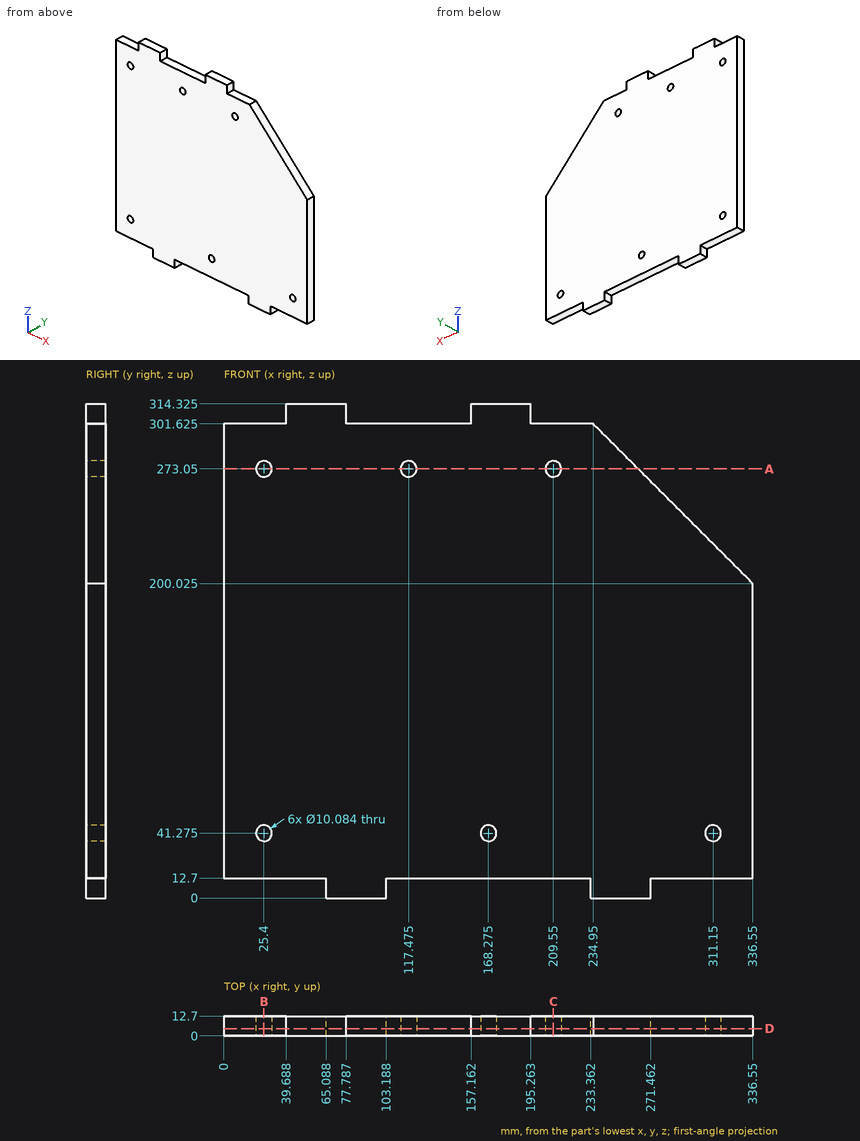
Here's the drawing with two shaded views (mm, measured from the low corner). I have some questions. Round coordinates to 2 decimals unless told otherwise and drop trailing zeros. Write each loop counter-clockwise with the first axis right and the second up, starting at its lowest first coordinate (ties: lowest second). Pieces come first, ordered by that corner, then holes. Notation, with made-up numbers: M -0.75,26 L 32.25,26 A14 cw 32.25,41 Z; hole C 80,17.5 d11. An arc over 180 degrees is marked long. Answer in a Markdown table with one row per item. Add a question column.
Q1. Imagine slicing it at D-D (y = 4.75). Give the number of separate pieces and of enclosed holes in the cut face, then the cut area to 3 significant figures.
Q2. Imagine slicing it at C-C (x = 209.55). Please give me the cut outline in (y, z) (1 decimal).
Q3. Will these pins go through, and if not, where does the flat tip stop? pin 1 Ø4 at (y, z) = (8.5, 3.5) entering from -X; pin 2 Ø4 at (y, z) = (9.5, 9) entering from +X; pin 3 Ø6 at (x, z) = (209.55, 273.05) entering from +Y; pin 4 Ø1.5 at (x, y) = (79, 10.5) entering from +Z (1 decimal).
Q4. Imagine slicing it at B-B (x = 25.4). Please give me the cut outline in (y, z) (1 decimal).
Q5. If I drill on line 1 (Z direction, x = 133.5, y = 9.25) (1 decimal); line 2 (X direction, y = 8.25, z = 273.05) (1 decimal); line 3 (Z direction, x = 311.15, y = 4.25) (1 decimal), over which ranges is the centre line in solid material (lowest first)? Write a range as from..to.
Q6. Imagine slicing it at A-A (z = 273.05). Please give me the cut outline in (x, y) (1 decimal).
Values:
| question | item | result |
|---|---|---|
| 1 | separate pieces | 1 |
| 1 | enclosed holes | 6 |
| 1 | area | 93,500 mm^2 |
| 2 | outline | M 0,12.7 L 12.7,12.7 L 12.7,268 L 0,268 Z; M 0,278.1 L 12.7,278.1 L 12.7,301.6 L 0,301.6 Z |
| 3 | pin 1 | x = 65.09 |
| 3 | pin 2 | x = 271.46 |
| 3 | pin 3 | through |
| 3 | pin 4 | z = 301.6 |
| 4 | outline | M 0,12.7 L 12.7,12.7 L 12.7,36.2 L 0,36.2 Z; M 0,46.3 L 12.7,46.3 L 12.7,268 L 0,268 Z; M 0,278.1 L 12.7,278.1 L 12.7,301.6 L 0,301.6 Z |
| 5 | line 1 | 12.7..301.6 |
| 5 | line 2 | 0..20.4, 30.4..112.4, 122.5..204.5, 214.6..263.5 |
| 5 | line 3 | 12.7..36.2, 46.3..225.4 |
| 6 | outline | M 0,0 L 20.4,0 L 20.4,12.7 L 0,12.7 Z; M 30.4,0 L 112.4,0 L 112.4,12.7 L 30.4,12.7 Z; M 122.5,0 L 204.5,0 L 204.5,12.7 L 122.5,12.7 Z; M 214.6,0 L 263.5,0 L 263.5,12.7 L 214.6,12.7 Z |
